Source: three-view drawing plus pictorial views. Frame: mm from the lowest corner of the part. Round coordinates to 2 decimals unless told otherwise and drop trailing zeros. Write each loop counter-clockwise with the first axis right and the second up, starting at its lowest first coordinate (ties: lowest second). Pieces come first, ordered by that corner, then holes. Notation, with made-up numbers: (33, -8) - (76, -8) arc R4 cw to (76, -4) - close; hole circle Ø8 at (5, 39.25). An arc over 180 degrees is marked (long way). Write each question's results on one line, items separated by ' | '.
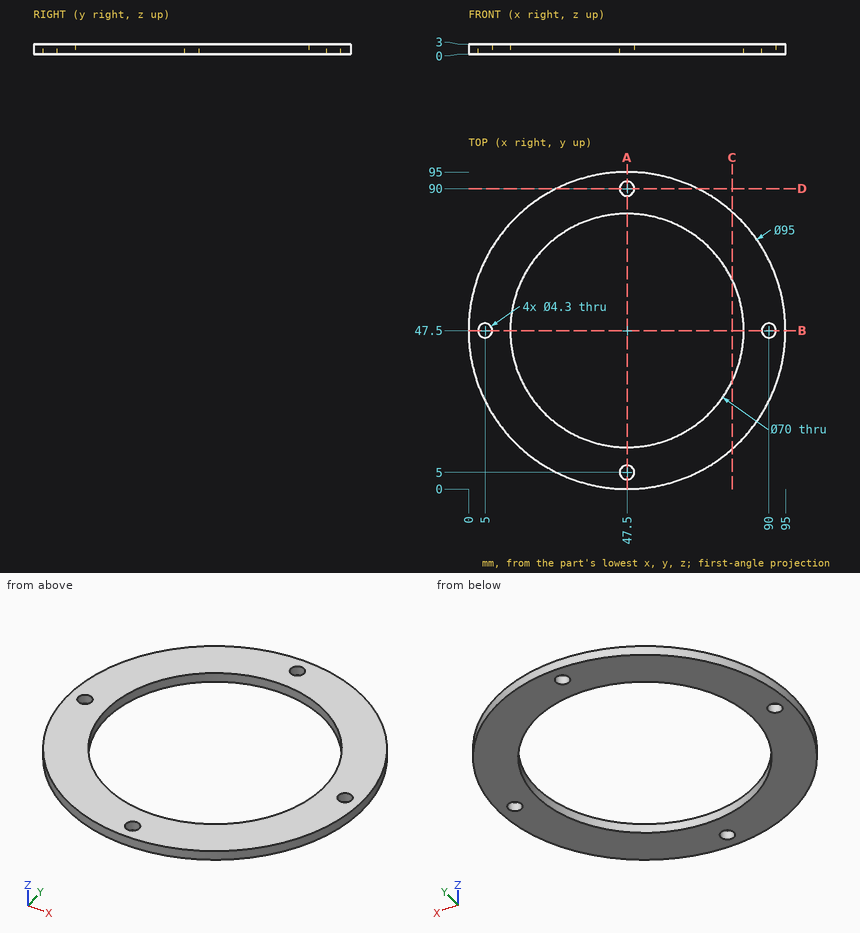
Q1. Section query D-D, the plane y = 90. Return loops of the section in (x, z).
Answer block:
outline: (26.29, 0) - (45.35, 0) - (45.35, 3) - (26.29, 3) - close; (49.65, 0) - (68.71, 0) - (68.71, 3) - (49.65, 3) - close
Q2. Section query C-C, the plane x = 79. Return loops of the section in (y, z), plus the area to 3 significant figures.
Answer block:
outline: (11.95, 0) - (32.24, 0) - (32.24, 3) - (11.95, 3) - close; (62.76, 0) - (83.05, 0) - (83.05, 3) - (62.76, 3) - close | area: 122 mm2
Q3. Pin query (flat end, axial travel): pin 1 (1 mm diameter, centred on x = 76.5, z = 1, fed in from -Y). Return the tip coordinate at first contact, or that it passes through.
Answer block:
pin 1: y = 9.5
Q4. Ray query, line 1 along Y through (x, z) = (47.5, 2.2); line 2 along Y through (x, z) = (54.5, 1.3); line 3 along X through (y, z) = (58, 1.7). Return the intervals inside material, ascending.
Answer block:
line 1: 0 to 2.85, 7.15 to 12.5, 82.5 to 87.85, 92.15 to 95 | line 2: 0.52 to 13.21, 81.79 to 94.48 | line 3: 1.18 to 14.11, 80.89 to 93.82
Q5. Section query A-A, the plane x = 47.5. Return loops of the section in (y, z).
Answer block:
outline: (0, 0) - (2.85, 0) - (2.85, 3) - (0, 3) - close; (7.15, 0) - (12.5, 0) - (12.5, 3) - (7.15, 3) - close; (82.5, 0) - (87.85, 0) - (87.85, 3) - (82.5, 3) - close; (92.15, 0) - (95, 0) - (95, 3) - (92.15, 3) - close
